```python
from build123d import *

# Parameters (mm, degrees)
SKETCH1_R      = 1.2
EXTRUDE1_DEPTH = 8
SKETCH2_R      = 1
EXTRUDE2_DEPTH = 1


with BuildPart() as part:
    # Sketch1 → Extrude1 (new body)
    with BuildSketch(Plane(origin=(0, 0, 0), x_dir=(1, 0, 0), z_dir=(0, 1, 0))):
        with BuildLine():
            Line((26.419805568, 30.469633485), (26.419805568, 25.969633485))
            Line((26.419805568, 25.969633485), (25.419805568, 25.969633485))
            Line((25.419805568, 25.969633485), (25.419805568, 23.469633485))
            Line((25.419805568, 23.469633485), (26.419805568, 23.469633485))
            Line((26.419805568, 23.469633485), (26.419805568, 18.469633485))
            Line((26.419805568, 18.469633485), (29.919805568, 18.469633485))
            Line((29.919805568, 18.469633485), (29.919805568, 23.469633485))
            Line((29.919805568, 23.469633485), (30.919805568, 23.469633485))
            Line((30.919805568, 23.469633485), (30.919805568, 25.969633485))
            Line((30.919805568, 25.969633485), (29.919805568, 25.969633485))
            Line((29.919805568, 25.969633485), (29.919805568, 30.469633485))
            Line((29.919805568, 30.469633485), (33.419805568, 30.469633485))
            Line((33.419805568, 30.469633485), (33.419805568, 12.969633485))
            ThreePointArc((33.419805568, 12.969633485), (32.541125911, 10.848313142), (30.419805568, 9.969633485))
            Line((30.419805568, 9.969633485), (12.919805568, 9.969633485))
            ThreePointArc((12.919805568, 9.969633485), (10.798485224, 10.848313142), (9.919805568, 12.969633485))
            Line((9.919805568, 12.969633485), (9.919805568, 30.469633485))
            Line((9.919805568, 30.469633485), (9.919805568, 37.969633485))
            Line((9.919805568, 37.969633485), (17.919805568, 37.969633485))
            Line((17.919805568, 37.969633485), (17.919805568, 30.469633485))
            Line((17.919805568, 30.469633485), (26.419805568, 30.469633485))
        make_face()
        with Locations(Location((23.169805568, 17.669633485, 0), (0, 0, 270))):
            Circle(SKETCH1_R, mode=Mode.SUBTRACT)
        with Locations(Location((13.669805568, 17.669633485, 0), (0, 0, 270))):
            Circle(SKETCH1_R, mode=Mode.SUBTRACT)
    extrude(amount=EXTRUDE1_DEPTH)

    # Sketch2 → Extrude2 (cut)
    with BuildSketch(Plane(origin=(0, 0, -18.469633485), x_dir=(-1, 0, 0), z_dir=(0, 0, -1))):
        with Locations((-28.169805568, 4)):
            Circle(SKETCH2_R)
    extrude(amount=-EXTRUDE2_DEPTH, mode=Mode.SUBTRACT)


solid = part.part
```
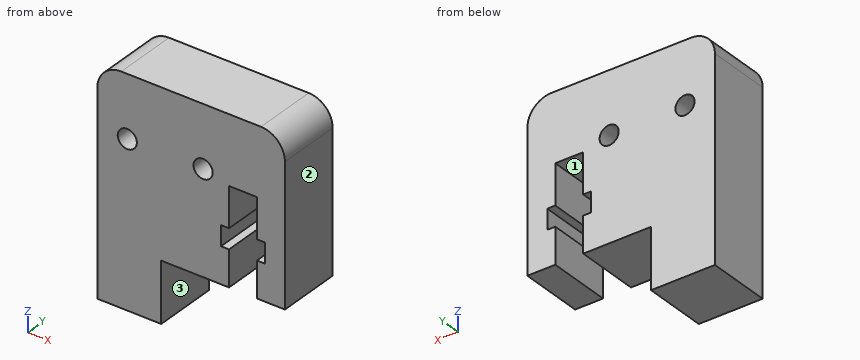
Verification items for the finished model (mm, model axes). Face numbers are marked on the shaded views. A direction names the side the tool comes from. Give positions to 0.01 mm unless a question says otherwise; leave off trailing zeros. Write each loop counter-clockwise with the first axis right and the second up, starting at its lowest first coordinate (ties: lowest second). Pieces come first, ordered by that corner, then holes. Notation, with made-up numbers: (8.5, 40.5) - (63.5, 40.5) arc R21 ccw to (63.5, 63.5) - close; hole circle Ø3 at (74, 77). An arc over 180 degrees is marked (long way). Put each result on its own line as item: value.
Q1. Set-up check for the marked faces 1, 2 and 3: record each of +Z, -Z, +X, -X, +Y, -Y from which the full face is reachable in a straight line by a thin tool's end or side.
Result:
face 1: -Z, +Y, -Y
face 2: +Z, -Z, +X, +Y, -Y
face 3: -Z, +X, +Y, -Y
Q2. Depth check by flat-ended pin: P1, Ø4, axis at x = 23, y = 3.5, coming from the -Z side; P2, Ø1.9, axis at x = 23.17, z = -17.67, coming from the +Y side. Enter the tip coordinate at first touch or a pass-through.
Result:
P1: z = -30.47
P2: through
Q3. Section check A-A on z = -19.5. Record the cut outline in (x, y), and give its area (3 significant figures).
Result:
outline: (9.92, 0) - (26.42, 0) - (26.42, 8) - (9.92, 8) - close; (29.92, 0) - (33.42, 0) - (33.42, 8) - (29.92, 8) - close
area: 160 mm2
Q4. Scan lines: probe 1 along X at (y, z) = (2, -29.75); probe 2 along X at (y, z) = (6.25, -25); probe 3 along Z at (x, y) = (30.5, 3). Record each from-to range of solid material in increasing order. Write a range as from..to.
Result:
probe 1: 9.92..26.42, 29.92..33.42
probe 2: 9.92..25.42, 30.92..33.42
probe 3: -30.47..-25.97, -23.47..-9.97
Q5. Section check B-B on y = 4. Record the cut outline in (x, z), and give its area (3 significant figures).
Result:
outline: (9.92, -37.97) - (17.92, -37.97) - (17.92, -30.47) - (26.42, -30.47) - (26.42, -25.97) - (25.42, -25.97) - (25.42, -23.47) - (26.42, -23.47) - (26.42, -18.47) - (27.17, -18.47) - (27.17, -17.47) - (29.17, -17.47) - (29.17, -18.47) - (29.92, -18.47) - (29.92, -23.47) - (30.92, -23.47) - (30.92, -25.97) - (29.92, -25.97) - (29.92, -30.47) - (33.42, -30.47) - (33.42, -12.97) arc R3 ccw to (30.42, -9.97) - (12.92, -9.97) arc R3 ccw to (9.92, -12.97) - close; hole circle Ø2.4 at (13.67, -17.67); hole circle Ø2.4 at (23.17, -17.67)
area: 480 mm2
Q6. Section check D-D on x = 21.5. Record the cut outline in (y, z).
Result:
outline: (0, -30.47) - (8, -30.47) - (8, -9.97) - (0, -9.97) - close
Q7. Section check C-C on z = -25.25. Record the cut outline in (x, y).
Result:
outline: (9.92, 0) - (25.42, 0) - (25.42, 8) - (9.92, 8) - close; (30.92, 0) - (33.42, 0) - (33.42, 8) - (30.92, 8) - close
